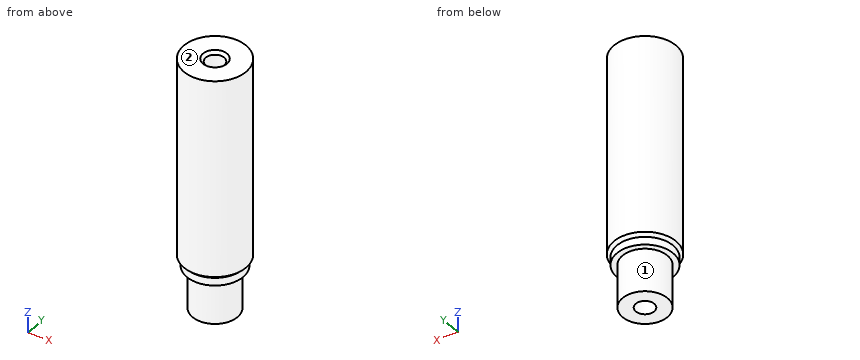
from build123d import *

# Parameters (mm, degrees)
CHAMFER_SIZE = 1


with BuildPart() as part:
    # Sketch → Revolution (revolve)
    with BuildSketch(Plane.XZ):
        Polygon((3.25, 70), (11, 70), (11, 0), (9.95, -1.05), (9.95, -3.8), (7.95, -3.8), (7.95, -19), (3.25, -19), align=None)
    revolve(axis=Axis((0, 0, 0), (0, 0, 1)))

    # Chamfer
    chamfer_edges = [part.edges().sort_by_distance(p)[0] for p in [
        (-3.25, 0, 70),
    ]]
    chamfer(chamfer_edges, length=CHAMFER_SIZE)


solid = part.part
Read the model definition and answer for the solid it produces. Units are mm, in the model's axes. Face numbers are marked on the shaded views. A direction names the side the tool comes from. Coordinates: 2 decimals unless noted, no trailing zeros. Loops run counter-clockwise (first coordinate to the right, second up) from the corner with the lowest first, then second, coordinate; pieces in that order, holes last. Notation, with made-up numbers: (1.25, 7) -> (5.25, 7) arc R27 cw to (5.25, 40) -> close; hole circle Ø9 at (23.25, -35). An arc over 180 degrees is marked (long way). Write item = value, one per line. Start each with the question number.
1) Given P1, Ø8, axis at x = -7, z = 26.5, coming from the +Y side; P2, Ø8, axis at x = 0.5, y = 3, coming from the +Z side; P3, Ø2, axis at x = 1.5, y = -1, coming from the -Z side; P4, Ø1, axis at x = -7, z = 29.5, coming from the -Y side, each flat-ended and moving along its own axis, determine where each tip first touches the part or whether it passes through.
2) The part is cut by section C-C, the plane z = 62.5. Determine the outline of the cut face in (x, y).
3) For the marked faces 1 and 2, determine the directions among +Z, -Z, +X, -X, +Y, -Y from which every point of the face is accessible in a straight line to the end or side of a thin tool.
4) The part is cut by section A-A, the plane x = 0. Determine the outline of the cut face in (y, z).
5) Find the intervals of material crossed by L1, parallel to Y at x = 0, z = 45.5; L2, parallel to Z at x = 0, y = -9.5; L3, parallel to Y at x = -3, z = 42, in increasing order. Write a range as from..to.
Result:
q1.P1 = 10.58
q1.P2 = 70
q1.P3 = through
q1.P4 = -8.87
q2.outline = circle Ø22 at (0, 0); hole circle Ø6.5 at (0, 0)
q3.face_1 = -Z
q3.face_2 = +Z, +X, -X, +Y, -Y
q4.outline = (-11, 0) -> (-9.95, -1.05) -> (-9.95, -3.8) -> (-7.95, -3.8) -> (-7.95, -19) -> (-3.25, -19) -> (-3.25, 69) -> (-4.25, 70) -> (-11, 70) -> close; (3.25, -19) -> (7.95, -19) -> (7.95, -3.8) -> (9.95, -3.8) -> (9.95, -1.05) -> (11, 0) -> (11, 70) -> (4.25, 70) -> (3.25, 69) -> close
q5.L1 = -11..-3.25, 3.25..11
q5.L2 = -3.8..70
q5.L3 = -10.58..-1.25, 1.25..10.58
